The listing builds one solid part. Answer for the finished solid, in the listing's coordinates (mm). A direction names the side the tool comes from. Give positions to 0.01 mm unless a question says otherwise; leave off trailing zeros. Write each loop counter-clockwise with the first axis right and the second up, starting at its lowest first coordinate (ties: lowest second). Pieces come first, ordered by that corner, then holes. Notation, with made-up numbers: (65, 32.25) -> (78, 32.25) arc R16 ccw to (78, 61.25) -> close; hole circle Ø9 at (40.5, 70). An arc over 180 degrees is marked (long way). Put each result on its own line as item: value. Start each with the question number.
1) For faces 1 (the cylindrical face through (6.768, -6.816, -0.74)), 2 (the flat face through (60, -55, 2)), 3 (the cylindrical face through (8.389, -103.694, 0.376)), determine the directions among +Z, -Z, +X, -X, +Y, -Y from which every point of the face is accessible in a straight line to the end or side of a thin tool.
2) A cutting plane is placed at D-D (x = 30). Write down the section's boundary in (y, z).
3) A cutting plane is placed at C-C (y = -49.5). Write down the section's boundary in (x, z).
4) Find the intervals of material crossed by line 1 along Y through (x, z) = (4.6, 1.45); line 2 along X through (y, z) = (-30, 2.6); line 3 along X through (y, z) = (-107.4, 1), in increasing order. Write a range as from..to.
5) Flat-ended cylindrical pins translate along their axes: pin 1 Ø10 at (x, y) = (18, -38.5) entering from -Z; pin 2 Ø3.5 at (x, y) = (4.6, -4.6) entering from +Z; pin 3 Ø0.8 at (y, z) = (-3.5, -0.5) entering from +X. Find the tip coordinate at first contact, or state that the pin passes through.
6) A cutting plane is placed at A-A (y = -30). Write down the section's boundary in (x, z), then the cut area to 3 significant figures.
7) A cutting plane is placed at B-B (x = 40). Write down the section's boundary in (y, z).
8) For a pull along Y with two mould halves and no side action, classify faces 4 (the flat face through (30, 0, 2)), 5 (the flat face through (57, -68, -1.5)), 6 (the cylindrical face through (4.53, -3, 1.21)), 7 (the cylindrical face through (6.959, -105.092, -0.74)) as released by +Y, released by -Y, zero draft, split by the parting line, or undercut.
Autodesk Fusion 360 part; units mm, degrees
sketch "Esquisse1" plane through (0, 0, 0) normal (0, 0, 1) x (1, 0, 0)
  line L0 (0, 0) -> (60, 0)
  line L1 (60, 0) -> (60, -112)
  line L2 (60, -112) -> (0, -112)
  line L3 (0, -112) -> (0, 0)
  dimension "d1" = 60
  dimension "d2" = 112
extrude "Extrusion1" add sketch "Esquisse1" along normal blind 4
sketch "Esquisse2" plane through (0, 0, 4) normal (0, 0, 1) x (-1, 0, 0)
  line L0 (0, 112) -> (-60, 112)
  line L1 (-60, 112) -> (-60, 0)
  line L2 (-60, 0) -> (0, 0)
  line L3 (0, 0) -> (0, 112)
  circle A0 centre (-4.6, 4.6) radius 1.6
  circle A1 centre (-4.6, 4.6) radius 1.6
  circle A2 centre (-55.4, 4.6) radius 1.6
  circle A3 centre (-4.6, 107.4) radius 1.6
  circle A4 centre (-55.4, 107.4) radius 1.6
  dimension "d5" = 3.2
  dimension "d6" = 4.6
  dimension "d7" = 4.6
  dimension "d8" = 3.2
  dimension "d9" = 3.2
  dimension "d10" = 4.6
  dimension "d11" = 4.6
  dimension "d12" = 3.2
  dimension "d13" = 4.6
  dimension "d14" = 4.6
  dimension "d15" = 3.2
  dimension "d16" = 4.6
  dimension "d17" = 4.6
hole "Perçage1" at (4.6, -4.6, 4) at (55.4, -4.6, 4) at (55.4, -107.4, 4) at (4.6, -107.4, 4) direction (0, 0, -1) diameter 3.2 depth 25 tip angle 118 countersink diameter 6.3 countersink angle 90
fillet "Congé1" radius 4.6 4 edges at (0, 0, 2) (60, 0, 2) (60, -112, 2) (0, -112, 2)
sketch "Esquisse3" plane through (0, 0, 0) normal (0, 0, -1) x (1, 0, 0)
  circle A0 centre (55.4, 107.4) radius 1.6
  circle A1 centre (4.6, 4.6) radius 1.6
  circle A2 centre (55.4, 4.6) radius 1.6
  circle A3 centre (4.6, 107.4) radius 1.6
  arc A4 (4.6, 112) -> (0, 107.4) centre (4.6, 107.4) ccw
  line L0 (0, 107.4) -> (0, 4.6)
  arc A5 (0, 4.6) -> (4.6, 0) centre (4.6, 4.6) ccw
  line L1 (4.6, 0) -> (55.4, 0)
  arc A6 (55.4, 0) -> (60, 4.6) centre (55.4, 4.6) ccw
  line L2 (60, 4.6) -> (60, 107.4)
  arc A7 (60, 107.4) -> (55.4, 112) centre (55.4, 107.4) ccw
  line L3 (55.4, 112) -> (4.6, 112)
  line L4 (8.9, 110) -> (51.6, 110)
  line L5 (2, 8.7) -> (2, 103.1)
  line L6 (52.1, 107.4) -> (52.1, 109.5)
  arc A8 (52.1, 107.4) -> (55.4467, 104.1003) centre (55.4, 107.4) ccw
  line L7 (55.3533, 104.1003) -> (57.5, 104.1003)
  arc A9 (52.1, 109.5) -> (51.6, 110) centre (51.6, 109.5) ccw
  arc A10 (58, 103.6003) -> (57.5, 104.1003) centre (57.5, 103.6003) ccw
  line L8 (7.9, 109) -> (7.9, 107.4)
  line L9 (3, 104.1) -> (4.6, 104.1)
  arc A11 (4.6, 104.1) -> (7.9, 107.4) centre (4.6, 107.4) ccw
  line L10 (3, 7.7) -> (4.6, 7.7)
  line L11 (7.7, 3) -> (7.7, 4.6)
  arc A12 (7.7, 4.6) -> (4.6, 7.7) centre (4.6, 4.6) ccw
  line L12 (57, 7.7) -> (55.4, 7.7)
  line L13 (52.3, 3) -> (52.3, 4.6)
  arc A13 (55.4, 7.7) -> (52.3, 4.6) centre (55.4, 4.6) ccw
  line L14 (58, 103.6003) -> (58, 8.7)
  line L15 (51.3, 2) -> (8.7, 2)
  arc A14 (8.9, 110) -> (7.9, 109) centre (8.9, 109) ccw
  arc A15 (3, 104.1) -> (2, 103.1) centre (3, 103.1) ccw
  arc A16 (2, 8.7) -> (3, 7.7) centre (3, 8.7) ccw
  arc A17 (7.7, 3) -> (8.7, 2) centre (8.7, 3) ccw
  arc A18 (51.3, 2) -> (52.3, 3) centre (51.3, 3) ccw
  arc A19 (57, 7.7) -> (58, 8.7) centre (57, 8.7) ccw
  line L16 (55.4592, 102.1003) -> (56, 102.1003)
  line L17 (56, 102.1003) -> (56, 9.7)
  line L18 (56, 9.7) -> (55.4, 9.7)
  arc A20 (55.4, 9.7) -> (50.3, 4.6) centre (55.4, 4.6) ccw
  line L19 (50.3, 4) -> (50.3, 4.6)
  line L20 (50.3, 4) -> (9.7, 4)
  line L21 (9.7, 4) -> (9.7, 4.6)
  arc A21 (9.7, 4.6) -> (4.6, 9.7) centre (4.6, 4.6) ccw
  line L22 (4, 9.7) -> (4.6, 9.7)
  line L23 (4, 9.7) -> (4, 102.1)
  line L24 (4, 102.1) -> (4.6, 102.1)
  arc A22 (4.6, 102.1) -> (9.9, 107.4) centre (4.6, 107.4) ccw
  line L25 (9.9, 108) -> (9.9, 107.4)
  line L26 (9.9, 108) -> (50.1, 108)
  line L27 (50.1, 107.4) -> (50.1, 108)
  arc A23 (50.1, 107.4) -> (55.4592, 102.1003) centre (55.4, 107.4) ccw
  dimension "d25" = 2
  dimension "d27" = 2
  dimension "d28" = 2
  dimension "d30" = 0.5
  dimension "d31" = 0.5
  dimension "d36" = 1
  dimension "d37" = 2
sketch "Esquisse5" plane through (0, 0, 0) normal (0, 0, -1) x (1, 0, 0)
  circle A0 centre (30, 82.0769) radius 6
  dimension "d42" = 12
extrude "Extrusion4" cut sketch "Esquisse5" against normal blind 9
chamfer "Chanfrein1" distance 1 angle 45 1 edges at (24.406, -84.2466, 0)
extrude "Extrusion2" add sketch "Esquisse3" along normal blind 1.5 contours L4 L5 L6 A8 L7 A9 A10 L8 L9 A11 L10 L11 A12 L12 L13 A13 L14 L15 A14 A15 A16 A17 A18 A19
extrude "Extrusion3" cut 1 faces at (29.8256, -30.6684, 0) along direction (0, 0, 1) blind 2.2
sketch "Esquisse6" plane through (0, 0, 4) normal (0, 0, 1) x (-1, 0, 0)
  circle A0 centre (-30, 82.0769) radius 6
  arc A1 (0, 107.4) -> (-4.6, 112) centre (-4.6, 107.4) ccw
  line L0 (-4.6, 112) -> (-55.4, 112)
  arc A2 (-55.4, 112) -> (-60, 107.4) centre (-55.4, 107.4) ccw
  line L1 (-60, 107.4) -> (-60, 4.6)
  arc A3 (-60, 4.6) -> (-55.4, 0) centre (-55.4, 4.6) ccw
  line L2 (-55.4, 0) -> (-4.6, 0)
  arc A4 (-4.6, 0) -> (0, 4.6) centre (-4.6, 4.6) ccw
  line L3 (0, 4.6) -> (0, 107.4)
  circle A5 centre (-55.4, 107.4) radius 3.15
  circle A6 centre (-4.6, 4.6) radius 3.15
  circle A7 centre (-55.4, 4.6) radius 3.15
  circle A8 centre (-4.6, 107.4) radius 3.15
  circle A9 centre (-20, 30) radius 3.5
  circle A10 centre (-40, 30) radius 3.5
  dimension "d52" = 7
  dimension "d53" = 30
  dimension "d54" = 7
  dimension "d55" = 30
  dimension "d56" = 20
  dimension "d57" = 20
extrude "Extrusion5" cut sketch "Esquisse6" against normal blind 20 contours A9 | A10
equation "d6 = 3 mm + ( 3.2 / 2 ) * 1 mm"
Reply:
1. face 1: -Z, -X, +Y
1. face 2: +Z, -Z, +X, +Y, -Y
1. face 3: -Z
2. outline: (-112, 0) -> (-110, 0) -> (-110, -1.5) -> (-108, -1.5) -> (-108, 2.2) -> (-89.08, 2.2) -> (-89.08, 0) -> (-88.08, 1) -> (-88.08, 4) -> (-112, 4) -> close; (-76.08, 1) -> (-75.08, 0) -> (-75.08, 2.2) -> (-4, 2.2) -> (-4, -1.5) -> (-2, -1.5) -> (-2, 0) -> (0, 0) -> (0, 4) -> (-76.08, 4) -> close
3. outline: (0, 0) -> (2, 0) -> (2, -1.5) -> (4, -1.5) -> (4, 2.2) -> (56, 2.2) -> (56, -1.5) -> (58, -1.5) -> (58, 0) -> (60, 0) -> (60, 4) -> (0, 4) -> close
4. line 1: y = -112..-109, -105.8..-102.1, -9.7..-6.2, -3..0
4. line 2: x = 0..16.5, 23.5..36.5, 43.5..60
4. line 3: x = 0..3, 6.2..9.9, 50.1..53.8, 57..60
5. pin 1: stops at z = 2.2
5. pin 2: stops at z = 2.6
5. pin 3: stops at x = 52.3
6. outline: (0, 0) -> (2, 0) -> (2, -1.5) -> (4, -1.5) -> (4, 2.2) -> (16.5, 2.2) -> (16.5, 4) -> (0, 4) -> close; (23.5, 2.2) -> (36.5, 2.2) -> (36.5, 4) -> (23.5, 4) -> close; (43.5, 2.2) -> (56, 2.2) -> (56, -1.5) -> (58, -1.5) -> (58, 0) -> (60, 0) -> (60, 4) -> (43.5, 4) -> close
6. area: 106 mm2
7. outline: (-112, 0) -> (-110, 0) -> (-110, -1.5) -> (-108, -1.5) -> (-108, 2.2) -> (-33.5, 2.2) -> (-33.5, 4) -> (-112, 4) -> close; (-26.5, 2.2) -> (-4, 2.2) -> (-4, -1.5) -> (-2, -1.5) -> (-2, 0) -> (0, 0) -> (0, 4) -> (-26.5, 4) -> close
8. face 4: released by +Y
8. face 5: zero draft
8. face 6: undercut
8. face 7: released by -Y
